Build history of the part. All positions in model axes, mm. A direction names the side the tool comes from. Coordinates: 2 decimals unless noted, no trailing zeros. Order: outer loops, then holes, each group sorted by start corner. A loop starts at its lowest first (then second) coordinate and runs counter-clockwise, first axis right, second up. Notation, with made-up numbers: (16.25, 59) - (28.25, 59) arc R26 ccw to (28.25, 80) - close; hole circle Ø1 at (56.25, 30.5). An arc over 180 degrees is marked (long way). One line per item, written item: value.
from build123d import *

# Parameters (mm, degrees)
SKETCH_1_W          = 6
SKETCH_1_H          = 3
EXTRUDE_1_DEPTH     = 30
SKETCH_4_W          = 5.1
SKETCH_4_H          = 2.5
CUT_EXTRUDE_1_DEPTH = 30
SKETCH_6_W          = 3
SKETCH_6_H          = 0.836449827
CUT_EXTRUDE_2_DEPTH = 0.5
SKETCH_8_W          = 1.62
SKETCH_8_H          = 0.4
CUT_EXTRUDE_3_DEPTH = 0.5


with BuildPart() as part:
    # 草圖1 → 填料-伸長1 (new body)
    with BuildSketch(Plane.XY):
        Rectangle(SKETCH_1_W, SKETCH_1_H)
    extrude(amount=EXTRUDE_1_DEPTH)

    # 草圖4 → 除料-伸長1 (cut)
    with BuildSketch(Plane.XY.offset(30)):
        with Locations((0, 0.25)):
            Rectangle(SKETCH_4_W, SKETCH_4_H)
    extrude(amount=-CUT_EXTRUDE_1_DEPTH, mode=Mode.SUBTRACT)

    # 草圖6 → 除料-伸長2 (cut)
    with BuildSketch(Plane(origin=(0, -1.5, 0), x_dir=(-1, 0, 0), z_dir=(0, -1, 0))):
        with Locations((-0.05, -29.581775087)):
            Rectangle(SKETCH_6_W, SKETCH_6_H)
    extrude(amount=-CUT_EXTRUDE_2_DEPTH, mode=Mode.SUBTRACT)

    # 草圖8 → 除料-伸長3 (cut)
    with BuildSketch(Plane(origin=(0, -1.5, 0), x_dir=(-1, 0, 0), z_dir=(0, -1, 0))):
        with Locations((0.076588476, -28.963550173)):
            Rectangle(SKETCH_8_W, SKETCH_8_H)
    extrude(amount=-CUT_EXTRUDE_3_DEPTH, mode=Mode.SUBTRACT)


solid = part.part
1. Band-saw the part on B-B, the plane z = 9. Give the cut face in (x, y), and give its area (3 significant figures).
Values found:
outline: (-3, -1.5) - (3, -1.5) - (3, 1.5) - (2.55, 1.5) - (2.55, -1) - (-2.55, -1) - (-2.55, 1.5) - (-3, 1.5) - close
area: 5.25 mm2
2. Two-plate mould, pull along X, no slides. Class faces 3 (the face through (2.7, -0.3, 30)), 4 (the face through (0, -1, 15)), 5 (the face through (-3, 0, 15)): pulls with the +X half, pulls with the -X half, needs draft (parallel to the pull), parting line crosses it, or undercut.
Values found:
face 3: needs draft
face 4: undercut
face 5: pulls with the -X half
3. Band-saw the part on D-D, the plane x = 1. Give the cut face in (y, z), and give its area (3 significant figures).
Values found:
outline: (-1.5, 0) - (-1, 0) - (-1, 29.16) - (-1.5, 29.16) - close
area: 14.6 mm2
4. Band-saw the part on A-A, the plane y = -0.5. Give the cut face in (x, z), and give its area (3 significant figures).
Values found:
outline: (-3, 0) - (-2.55, 0) - (-2.55, 30) - (-3, 30) - close; (2.55, 0) - (3, 0) - (3, 30) - (2.55, 30) - close
area: 27.0 mm2
5. 3-axis set-ups, long thin cutter, end or side, ignore diameter. For faces 1 (the face through (2.55, 0, 15)), 2 (the face through (3, 0, 15)): which of +Z, -Z, +X, -X, +Y, -Y reach the whole face in a straight line?
Values found:
face 1: +Z, -Z, +Y
face 2: +Z, -Z, +X, +Y, -Y
6. Band-saw the part on C-C, the plane x = -0.15. Give the cut face in (y, z).
Values found:
outline: (-1.5, 0) - (-1, 0) - (-1, 28.76) - (-1.5, 28.76) - close
7. Probe line 1 along X through (y, z) = (-0.4, 17.5); line 2 along Y through (x, z) = (1.7, 28.5). List the from-to ranges inside material, lowest first.
Values found:
line 1: x = -3 to -2.55, 2.55 to 3
line 2: y = -1.5 to -1
